```python
from build123d import *

# Parameters (mm, degrees)
F0_W     = 26
F0_H     = 35
F0_R     = 1
F0_R_2   = 3
F1_DEPTH = 7
F2_W     = 30
F2_H     = 15
F3_DEPTH = 3
F5_DEPTH = 26


with BuildPart() as f1:
    # F0 (on Front) → F1 (new body)
    with BuildSketch(Plane.XZ):
        with Locations((0, 17.5)):
            Rectangle(F0_W, F0_H)
        with Locations((-7.707626, 17.128522)):
            Circle(F0_R, mode=Mode.SUBTRACT)
        with Locations((7.707626, 17.128522)):
            Circle(F0_R, mode=Mode.SUBTRACT)
        with Locations((0, 21.578522)):
            Circle(F0_R_2, mode=Mode.SUBTRACT)
        with Locations((0, 30.478522)):
            Circle(F0_R, mode=Mode.SUBTRACT)
    extrude(amount=F1_DEPTH)

    # F2 (on Top) → F3 (join)
    with BuildSketch(Plane.XY):
        with Locations((0, -5.5)):
            Rectangle(F2_W, F2_H)
    extrude(amount=-F3_DEPTH)

    # F4 (on face) → F5 (join)
    with BuildSketch(Plane(origin=(-13, 0, 0), x_dir=(0, -1, 0), z_dir=(-1, 0, 0))):
        Polygon((13.13559, 0), (7, 8.883364), (7, 6.872926), (11.747014, 0), align=None)
        Polygon((11.747014, 0), (7, 6.872926), (7, 4.174094), (9.882976, 0), align=None)
        Polygon((9.882976, 0), (7, 4.174094), (7, 1.96276), (8.355645, 0), align=None)
        Polygon((8.355645, 0), (7, 1.96276), (7, 0), align=None)
        Polygon((0, 4.22952), (0, 8.883364), (-1.634174, 0), (-0.778058, 0), align=None)
        Polygon((0, 0), (0, 4.22952), (-0.778058, 0), align=None)
    extrude(amount=-F5_DEPTH)


solid = f1.part
```
Check sheet for the modelled part. Datum: model origin and axes. Units: mm. A direction names the side the tool comes from. Coordinates: 2 decimals unless noted, no trailing zeros. Write each loop counter-clockwise with the first axis right and the second up, starting at its lowest first coordinate (ties: lowest second). Pieces come first, ordered by that corner, then holes. Notation, with made-up numbers: (23.25, 80) -> (45.25, 80) arc R32 ccw to (45.25, 111) -> close; hole circle Ø4 at (43.25, 47.5). An arc over 180 degrees is marked (long way). Use a Markdown table: item, result.
1. Sectioned sample at C-C (z = 31). Enter the section's corners in (x, y).
Reported:
| item | result |
|---|---|
| outline | (-13, -7) -> (-0.85, -7) -> (-0.85, 0) -> (-13, 0) -> close; (0.85, -7) -> (13, -7) -> (13, 0) -> (0.85, 0) -> close |
2. Sectioned sample at A-A (x = 0). Enter the section's corners in (y, z).
Reported:
| item | result |
|---|---|
| outline | (-13.14, 0) -> (-13, 0) -> (-13, -3) -> (2, -3) -> (2, 0) -> (1.63, 0) -> (0, 8.88) -> (0, 18.58) -> (-7, 18.58) -> (-7, 8.88) -> close; (-7, 24.58) -> (0, 24.58) -> (0, 29.48) -> (-7, 29.48) -> close; (-7, 31.48) -> (0, 31.48) -> (0, 35) -> (-7, 35) -> close |
3. Sectioned sample at B-B (x = 12.5). Enter the section's corners in (y, z), plus the area to 3 significant figures.
Reported:
| item | result |
|---|---|
| outline | (-13.14, 0) -> (-13, 0) -> (-13, -3) -> (2, -3) -> (2, 0) -> (1.63, 0) -> (0, 8.88) -> (0, 35) -> (-7, 35) -> (-7, 8.88) -> close |
| area | 325 mm2 |
4. Scan lines: line 1 along Z through (x, y) = (0, -1.75); line 2 along X through (y, z) = (-9, 4.5); line 3 along Y through (x, z) = (1, 28.5). Record each from-to range of solid material in increasing order.
Reported:
| item | result |
|---|---|
| line 1 | z = -3 to 18.58, 24.58 to 29.48, 31.48 to 35 |
| line 2 | x = -13 to 13 |
| line 3 | y = -7 to 0 |
5. Sectioned sample at D-D (y = -11.5). Enter the section's corners in (x, z), plus the area to 3 significant figures.
Reported:
| item | result |
|---|---|
| outline | (-15, -3) -> (15, -3) -> (15, 0) -> (13, 0) -> (13, 2.37) -> (-13, 2.37) -> (-13, 0) -> (-15, 0) -> close |
| area | 152 mm2 |
6. Tool access check on faces 1 (the flat face through (0, 0, 25)), 2 (the flat face through (13, -4, 14)), 3 (the flat face through (-0.1, 1.8, 0)). Record the directions out of +Z, -Z, +X, -X, +Y, -Y that give a thin tool (end or side, any length) a straight path to the whole face; none if there is none.
Reported:
| item | result |
|---|---|
| face 1 | +Z, +X, -X, +Y |
| face 2 | +Z, +X, +Y, -Y |
| face 3 | +Z, +Y |
7. Go/stop test with flat-tipped pins: pin 1 Ø6 at (x, z) = (0.5, 3.5) entering from +Y; pin 2 Ø2 at (x, z) = (10, 21.5) entering from +Y; pin 3 Ø3.5 at (x, z) = (-7, -2) entering from -Y. Record where each tip stops, or that it passes through.
Reported:
| item | result |
|---|---|
| pin 1 | stops at y = 1.54 |
| pin 2 | stops at y = 0 |
| pin 3 | stops at y = -13 |
